from build123d import *

# Parameters (mm, degrees)
F5_W     = 93.8750132918
F5_H     = 62.5833421946
F7_R     = 22.6051057699
F8_DEPTH = 93.98


# Not quite as in the source:
# - the arcs of a loft's sections are written as splines that run evenly, so that the points pair up as in the source's solid
# - the program builds the solid bodies; features that only make, move or delete a surface that nothing else refers to are left out


with BuildPart() as f6:
    # F5 (on Top) → F6 section 0
    with BuildSketch(Plane.XY):
        Rectangle(F5_W, F5_H)
    # F4 (on offset) → F6 section 1
    with BuildSketch(Plane.XY.offset(101.6)):
        with BuildLine():
            add(Edge.make_bspline(
                [(22.5525184305, 15.035012287), (21.5684791775, 16.5110711666), (20.439088741, 17.8901765373), (17.9328967072, 20.4016171121), (16.5561570804, 21.5338902158), (13.6081630734, 23.5081403532), (12.0369815881, 24.3500685697), (8.7604753642, 25.7112589441), (7.0552316437, 26.2304874441), (3.5761274997, 26.9263082729), (1.8023531039, 27.1028833962), (-1.7456489391, 27.1065946751), (-3.519788855, 26.9337307389), (-7.0003410682, 26.2451898455), (-8.706667302, 25.7295299139), (-11.9860140158, 24.3751970887), (-13.5589534074, 23.5365576836), (-15.035012287, 22.5525184305)],
                knots=[0, 0, 0, 0, 0.125, 0.125, 0.25, 0.25, 0.375, 0.375, 0.5, 0.5, 0.625, 0.625, 0.75, 0.75, 0.875, 0.875, 1, 1, 1, 1], degree=3))
            add(Edge.make_bspline(
                [(-15.035012287, 22.5525184305), (-16.5110711666, 21.5684791775), (-17.8901765373, 20.439088741), (-20.4016171121, 17.9328967072), (-21.5338902158, 16.5561570804), (-23.5081403532, 13.6081630734), (-24.3500685697, 12.0369815881), (-25.7112589441, 8.7604753642), (-26.2304874441, 7.0552316437), (-26.9263082729, 3.5761274997), (-27.1028833962, 1.8023531039), (-27.1065946751, -1.7456489391), (-26.9337307389, -3.519788855), (-26.2451898455, -7.0003410682), (-25.7295299139, -8.706667302), (-24.3751970887, -11.9860140158), (-23.5365576836, -13.5589534074), (-22.5525184305, -15.035012287)],
                knots=[0, 0, 0, 0, 0.125, 0.125, 0.25, 0.25, 0.375, 0.375, 0.5, 0.5, 0.625, 0.625, 0.75, 0.75, 0.875, 0.875, 1, 1, 1, 1], degree=3))
            add(Edge.make_bspline(
                [(-22.5525184305, -15.035012287), (-21.5684791775, -16.5110711666), (-20.439088741, -17.8901765373), (-17.9328967072, -20.4016171121), (-16.5561570804, -21.5338902158), (-13.6081630734, -23.5081403532), (-12.0369815881, -24.3500685697), (-8.7604753642, -25.7112589441), (-7.0552316437, -26.2304874441), (-3.5761274997, -26.9263082729), (-1.8023531039, -27.1028833962), (1.7456489391, -27.1065946751), (3.519788855, -26.9337307389), (7.0003410682, -26.2451898455), (8.706667302, -25.7295299139), (11.9860140158, -24.3751970887), (13.5589534074, -23.5365576836), (15.035012287, -22.5525184305)],
                knots=[0, 0, 0, 0, 0.125, 0.125, 0.25, 0.25, 0.375, 0.375, 0.5, 0.5, 0.625, 0.625, 0.75, 0.75, 0.875, 0.875, 1, 1, 1, 1], degree=3))
            add(Edge.make_bspline(
                [(15.035012287, -22.5525184305), (16.5110711666, -21.5684791775), (17.8901765373, -20.439088741), (20.4016171121, -17.9328967072), (21.5338902158, -16.5561570804), (23.5081403532, -13.6081630734), (24.3500685697, -12.0369815881), (25.7112589441, -8.7604753642), (26.2304874441, -7.0552316437), (26.9263082729, -3.5761274997), (27.1028833962, -1.8023531039), (27.1065946751, 1.7456489391), (26.9337307389, 3.519788855), (26.2451898455, 7.0003410682), (25.7295299139, 8.706667302), (24.3751970887, 11.9860140158), (23.5365576836, 13.5589534074), (22.5525184305, 15.035012287)],
                knots=[0, 0, 0, 0, 0.125, 0.125, 0.25, 0.25, 0.375, 0.375, 0.5, 0.5, 0.625, 0.625, 0.75, 0.75, 0.875, 0.875, 1, 1, 1, 1], degree=3))
        make_face()
    loft(ruled=True)

    # F7 (on offset) → F8 (cut)
    with BuildSketch(Plane.XY.offset(101.6)):
        Circle(F7_R)
    extrude(amount=-F8_DEPTH, mode=Mode.SUBTRACT)


solid = f6.part
Work out the finished part from the listing and answer in its coordinate system (mm). A direction names the side the tool comes from. Give positions to 0.01 mm unless a question says otherwise; leave off trailing zeros. Answer as CSV lines item,"result". Start each with the question number.
Q1. Find the intervals of material crossed by L1, parallel to Z at x = 9.5, y = 10.5; L2, parallel to Y at x = 0, z = 64; L3, parallel to Y at x = 0, z = 71, in increasing order. Write a range as [from, to].
Q2. The mould has two halves that part along X. Classify faces 1 (the face through (-2.943, 22.413, 55.268)), 2 (the face through (22, 7, 101.6)): +X half, -X half, draft (parallel to the pull), parting line (faces both ways), or undercut.
Q3. Given pin 1 Ø5 at (y, z) = (16.5, 17) entering from +X; pin 2 Ø10 at (y, z) = (-20, 20) entering from -X; pin 3 Ø1 at (x, z) = (-13.5, 85.5) entering from -Y, each flat-ended and moving along its own axis, determine where each tip first touches the part or whether it passes through.
Q4. For faces 3 (the face through (0, 0, 7.62)), 4 (the face through (-1, 0, 0)), determine the directions among +Z, -Z, +X, -X, +Y, -Y from which every point of the face is accessible in a straight line to the end or side of a thin tool.
Check result:
1,L1,"z = [0, 7.62]"
1,L2,"y = [-28.55, -22.61], [22.61, 28.55]"
1,L3,"y = [-28.28, -22.61], [22.61, 28.28]"
2,face 1,"undercut"
2,face 2,"draft"
3,pin 1,"stops at x = 43.98"
3,pin 2,"stops at x = -43.78"
3,pin 3,"stops at y = -25.27"
4,face 3,"+Z"
4,face 4,"-Z, +X, -X, +Y, -Y"
